```python
from build123d import *

# Parameters (mm, degrees)
SKETCH1_W           = 152.4
SKETCH1_H           = 12.7
SKETCH1_R           = 3.175
BOSS_EXTRUDE1_DEPTH = 2.54
FILLET2_R           = 6.35
FILLET3_R           = 6.35


with BuildPart() as part:
    # Sketch1 → Boss-Extrude1 (new body)
    with BuildSketch(Plane.XY):
        with Locations((76.2, 6.35)):
            Rectangle(SKETCH1_W, SKETCH1_H)
        with Locations((6.35, 6.35)):
            Circle(SKETCH1_R, mode=Mode.SUBTRACT)
        with Locations((146.05, 6.35)):
            Circle(SKETCH1_R, mode=Mode.SUBTRACT)
    extrude(amount=BOSS_EXTRUDE1_DEPTH)

    # Fillet2
    fillet2_edges = [part.edges().sort_by_distance(p)[0] for p in [
        (0, 0, 1.27),
        (0, 12.7, 1.27),
    ]]
    fillet(fillet2_edges, radius=FILLET2_R - 0.0001)  # a hair under: the kernel refuses the full size

    # Fillet3
    fillet3_edges = [part.edges().sort_by_distance(p)[0] for p in [
        (152.4, 0, 1.27),
        (152.4, 12.7, 1.27),
    ]]
    fillet(fillet3_edges, radius=FILLET3_R - 0.0001)  # a hair under: the kernel refuses the full size


solid = part.part
```
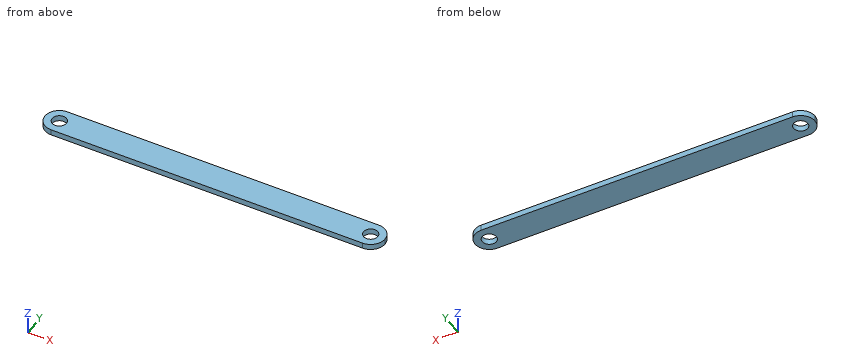
Could you check a few things on this model? Use its own coordinates, in mm. Round coordinates to 2 decimals unless told otherwise and drop trailing zeros. Loops run counter-clockwise (first coordinate to the right, second up) from the corner with the lowest first, then second, coordinate; pieces in that order, holes last. Notation, with made-up numbers: M 71.5,-4 L 103.5,-4 A4 ccw 103.5,1 Z; hole C -10.5,-38 d7. An arc over 180 degrees is marked long. Put each result on its own line as item: value.
Q1. Imagine slicing it at A-A (z = 0.7). State how many separate pieces and enclosed holes the cut face has, then the cut area to 3 significant figures.
Check result:
separate pieces: 1
enclosed holes: 2
area: 1,840 mm2
Q2. I need wall thicknesses on probe 1 along Y at (x, z) = (146.05, 1.35) (3 decimals); probe 2 along X at (y, z) = (9, 1.25); probe 3 along X at (y, z) = (9.25, 2.1). Which ranges of each line are inside material? Lowest first, please.
Check result:
probe 1: 0 to 3.175, 9.525 to 12.7
probe 2: 0.58 to 4.6, 8.1 to 144.3, 147.8 to 151.82
probe 3: 0.7 to 5.06, 7.64 to 144.76, 147.34 to 151.7
Q3. Imagine slicing it at C-C (y = 1.5). Write out the boundary of the cut face in (x, z), then the cut area to 3 significant figures.
Check result:
outline: M 2.25,0 L 150.15,0 L 150.15,2.54 L 2.25,2.54 Z
area: 376 mm2
Q4. Imagine slicing it at B-B (y = 8). Write out the boundary of the cut face in (x, z), then the cut area to 3 significant figures.
Check result:
outline: M 0.22,0 L 3.64,0 L 3.64,2.54 L 0.22,2.54 Z; M 9.06,0 L 143.34,0 L 143.34,2.54 L 9.06,2.54 Z; M 148.76,0 L 152.18,0 L 152.18,2.54 L 148.76,2.54 Z
area: 358 mm2
Q5. For pin 1 (4 mm diameter, centred on x = 146.05, y = 6.35, fed in from -Z); pin 2 (1 mm diameter, centred on y = 9, z = 2, fed in from +X) (3 decimals); pin 3 (1.5 mm diameter, centred on y = 9.5, z = 1, fed in from -X), each with a flat end and sliding along its axis, tell me the tip position at first contact or that it passes through.
Check result:
pin 1: through
pin 2: x = 152.025
pin 3: x = 0.47
